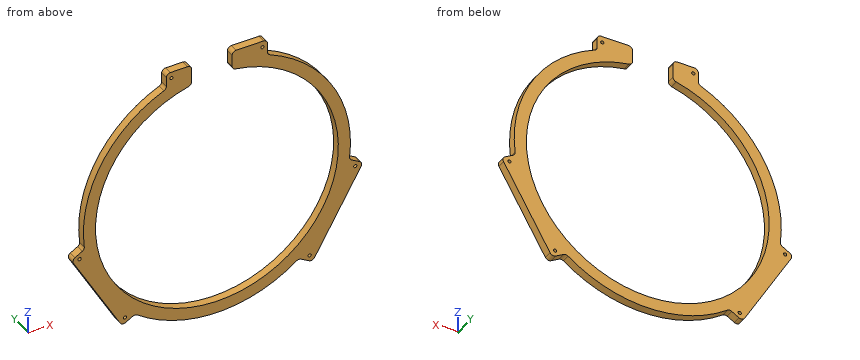
```python
from build123d import *

# Parameters (mm, degrees)
SKETCH1_R           = 1.6
BOSS_EXTRUDE2_DEPTH = 8


with BuildPart() as part:
    # Sketch1 → Boss-Extrude2 (new body)
    with BuildSketch(Plane(origin=(0, 0, 0), x_dir=(1, 0, 0), z_dir=(0, 1, 0))):
        with BuildLine():
            Line((-75.004193667, 160.867236212), (-67.830157516, 156.725304509))
            ThreePointArc((-67.830157516, 156.725304509), (-65.599707636, 156.196050035), (-63.444946383, 156.978367686))
            ThreePointArc((-63.444946383, 156.978367686), (15.265708014, 183.014099207), (93.976880337, 156.979933523))
            ThreePointArc((93.976880337, 156.979933523), (96.133483562, 156.197553795), (98.365264281, 156.728788517))
            Line((98.365264281, 156.728788517), (106.307271021, 161.324010437))
            ThreePointArc((106.307271021, 161.324010437), (109.343075496, 161.726207543), (111.773674482, 159.863397867))
            Line((111.773674482, 159.863397867), (157.816436501, 80.200975925))
            ThreePointArc((157.816436501, 80.200975925), (158.217214787, 77.164984073), (156.353269729, 74.735255986))
            Line((156.353269729, 74.735255986), (148.364199487, 70.122764131))
            ThreePointArc((148.364199487, 70.122764131), (146.790626728, 68.45576511), (146.390753061, 66.198528301))
            ThreePointArc((146.390753061, 66.198528301), (129.583526562, -14.983904944), (67.683015931, -70.132768158))
            ThreePointArc((67.683015931, -70.132768158), (65.928218191, -71.607690224), (65.271379414, -73.803885351))
            Line((65.271379414, -73.803885351), (65.271379414, -83.002595828))
            ThreePointArc((65.271379414, -83.002595828), (64.099806539, -85.831022953), (61.271379414, -87.002595828))
            Line((61.271379414, -87.002595828), (34.271379414, -87.002595828))
            ThreePointArc((34.271379414, -87.002595828), (31.44295229, -85.831022953), (30.271379414, -83.002595828))
            Line((30.271379414, -83.002595828), (30.271379414, -71.520933984))
            ThreePointArc((30.271379414, -71.520933984), (31.233931861, -68.918259905), (33.658335594, -67.568190978))
            ThreePointArc((33.658335594, -67.568190978), (20.194853463, 170.912875133), (-12.793277309, -65.659032482))
            ThreePointArc((-12.793277309, -65.659032482), (-10.586855707, -67.072391843), (-9.728620586, -69.548136872))
            Line((-9.728620586, -69.548136872), (-9.728620586, -83.002595828))
            ThreePointArc((-9.728620586, -83.002595828), (-10.900193461, -85.831022953), (-13.728620586, -87.002595828))
            Line((-13.728620586, -87.002595828), (-30.728620586, -87.002595828))
            ThreePointArc((-30.728620586, -87.002595828), (-33.55704771, -85.831022953), (-34.728620586, -83.002595828))
            Line((-34.728620586, -83.002595828), (-34.728620586, -73.807656468))
            ThreePointArc((-34.728620586, -73.807656468), (-35.38553605, -71.611344607), (-37.140513481, -70.136428359))
            ThreePointArc((-37.140513481, -70.136428359), (-99.047180019, -14.987896579), (-115.856711089, 66.198528301))
            ThreePointArc((-115.856711089, 66.198528301), (-116.256584757, 68.45576511), (-117.830157516, 70.122764131))
            Line((-117.830157516, 70.122764131), (-125.004193667, 74.264695834))
            ThreePointArc((-125.004193667, 74.264695834), (-126.867896972, 76.693521268), (-126.468295282, 79.728797449))
            Line((-126.468295282, 79.728797449), (-80.468295282, 159.403134597))
            ThreePointArc((-80.468295282, 159.403134597), (-78.039469847, 161.266837902), (-75.004193667, 160.867236212))
        make_face()
        with Locations(Location((-75.598775183, 155.43701163, 0), (0, 0, 270))):
            Circle(SKETCH1_R, mode=Mode.SUBTRACT)
        with Locations(Location((-120.526355361, 77.452098276, 0), (0, 0, 270))):
            Circle(SKETCH1_R, mode=Mode.SUBTRACT)
        with Locations(Location((106.909257313, 155.885291293, 0), (0, 0, 270))):
            Circle(SKETCH1_R, mode=Mode.SUBTRACT)
        with Locations(Location((151.982456893, 77.984449703, 0), (0, 0, 270))):
            Circle(SKETCH1_R, mode=Mode.SUBTRACT)
        with Locations(Location((-29.728620586, -80.802595828, 0), (0, 0, 270))):
            Circle(SKETCH1_R, mode=Mode.SUBTRACT)
        with Locations(Location((60.271379414, -80.802595828, 0), (0, 0, 270))):
            Circle(SKETCH1_R, mode=Mode.SUBTRACT)
    extrude(amount=BOSS_EXTRUDE2_DEPTH)


solid = part.part
```
Could you check a few things on this model? Use its own coordinates, in mm. Round coordinates to 2 decimals unless told otherwise and drop trailing zeros. Loops run counter-clockwise (first coordinate to the right, second up) from the corner with the lowest first, then second, coordinate; pieces in that order, holes last. Notation, with made-up numbers: (52, 1.5) - (96, 1.5) arc R29 ccw to (96, 21.5) - close; hole circle Ø11 at (48.25, 82). An arc over 180 degrees is marked (long way). Answer as CSV lines item,"result".
1. For pin 1 Ø3 at (x, y) = (12, 4.5) entering from +Z; pin 2 Ø1.5 at (y, z) = (4.5, 10.5) entering from -X, each with a flat end and sliding along its axis, tell me the tip position at first contact or that it passes through.
Filled in:
pin 1,"stops at z = -170.92"
pin 2,"stops at x = -101.92"
2. I want a section at A-A on z = -86. List the corners of the cut face in (x, y) for me.
Filled in:
outline,"(-122.85, 0) - (-99.52, 0) - (-99.52, 8) - (-122.85, 8) - close; (130.05, 0) - (154.46, 0) - (154.46, 8) - (130.05, 8) - close"
3. I want a section at D-D on y = 3.5. Count the separate pieces of the cut face and the enclosed holes in it, then the cut area to 3 significant figures.
Filled in:
separate pieces,"1"
enclosed holes,"6"
area,"11,400 mm^2"
4. I want a section at C-C on x = -2.5. List the corners of the cut face in (y, z) for me.
Filled in:
outline,"(0, -181.81) - (8, -181.81) - (8, -169.69) - (0, -169.69) - close"
5. Please list where these lines run through material, in increasing order: line 1 along Z through (x, y) = (-76.5, 5); line 2 along X through (y, z) = (7.5, -50); line 3 along Z through (x, y) = (51, 5.75). Write a range as [from, to].
Filled in:
line 1,"z = [-161.37, -156.76], [-154.11, -128.34], [26.31, 43.87]"
line 2,"x = [-116.73, -104.73], [135.26, 147.26]"
line 3,"z = [-178.09, -165.57], [63.54, 87]"
6. I want a section at B-B on x = 73. List the corners of the cut face in (y, z) for me.
Filled in:
outline,"(0, -169.72) - (8, -169.72) - (8, -156.21) - (0, -156.21) - close; (0, 54.19) - (8, 54.19) - (8, 67.69) - (0, 67.69) - close"
